Input: part model. Units: mm. Frame: model coordinates. Face numbers are marked on the shaded views. A direction names the side the tool comes from. Coordinates: 2 decimals unless noted, no trailing zeros. Order: outer loops, then holes, each group sorted by start corner. A loop starts at its lowest first (then second) coordinate and runs counter-clockwise, first axis right, second up.
Autodesk Inventor part; units mm, degrees
ref_plane "YZ Plane" through (0, 0, 0) normal (1, 0, 0) x (0, 1, 0)
ref_plane "XZ Plane" through (0, 0, 0) normal (0, 1, 0) x (-1, 0, 0)
ref_plane "XY Plane" through (0, 0, 0) normal (0, 0, 1) x (1, 0, 0)
sketch "Sketch1" plane through (0, 0, 0) normal (0, 1, 0) x (-1, 0, 0)
  line L0 (14.4237, 0) -> (-15, 0)
  line L1 (0, 25) -> (0, -25.6825)
  line L2 (6.5, 6.5) -> (-6.5, 6.5)
  line L3 (-6.5, 6.5) -> (-6.5, -6.5)
  line L4 (-6.5, -6.5) -> (6.5, -6.5)
  line L5 (6.5, -6.5) -> (6.5, 6.5)
  point P0 (0, 0)
  dimension "d0" = 13
  dimension "d1" = 0
  dimension "d10" = 0
extrude "Body" add sketch "Sketch1" along normal blind 20
sketch "Sketch2" plane through (0, 0, 0) normal (0, -1, 0) x (1, 0, 0)
  circle A0 centre (0, 0) radius 2.6
  dimension "d4" = 5.2
extrude "Screw Thread Hole" cut sketch "Sketch2" against normal through all
sketch "Sketch3" plane through (0, 20, 0) normal (0, 1, 0) x (1, 0, 0)
  line L0 (4.25, -4.25) -> (-4.25, -4.25)
  line L1 (-4.25, -4.25) -> (-4.25, 4.25)
  line L2 (-4.25, 4.25) -> (4.25, 4.25)
  line L3 (4.25, 4.25) -> (4.25, -4.25)
  line L4 (4.25, -4.25) -> (-4.25, 4.25) construction
  line L5 (-4.25, -4.25) -> (4.25, 4.25) construction
  point P0 (0, 0)
  dimension "d11" = 8.5
extrude "Connector" cut sketch "Sketch3" against normal blind 6
properties part number "Screw Port 6_8"
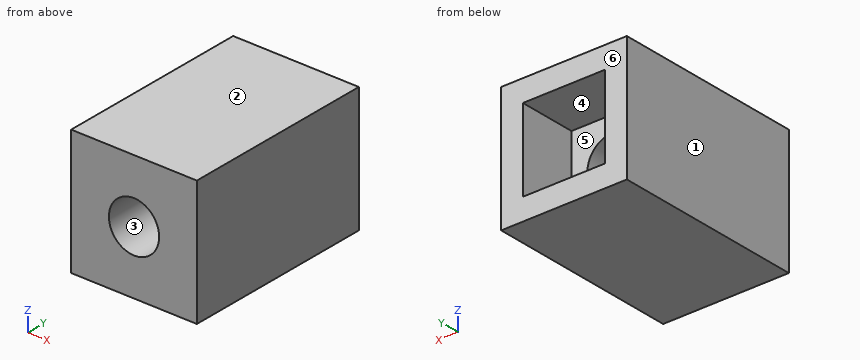
Item 1: Pin query (flat end, axial travel): pin 1 Ø4 at (x, z) = (-1.5, 0) entering from +Y. Return the tip coordinate at first contact, or that it passes through.
Response values:
pin 1: stops at y = 14
Item 2: Cut plane C-C on x = 0. Return loops of the section in (y, z), then the cut area to 3 significant figures.
Response values:
outline: (0, -6.5) - (20, -6.5) - (20, -4.25) - (14, -4.25) - (14, -2.6) - (0, -2.6) - close; (0, 2.6) - (14, 2.6) - (14, 4.25) - (20, 4.25) - (20, 6.5) - (0, 6.5) - close
area: 136 mm2
Item 3: Ray query, probe 1 along Z at (x, y) = (-1.75, 18); probe 2 along Z at (x, y) = (0, 6.25). Return the intervals inside material, ascending.
Response values:
probe 1: z = -6.5 to -4.25, 4.25 to 6.5
probe 2: z = -6.5 to -2.6, 2.6 to 6.5
Item 4: Cut plane D-D on x = 3.5. Return loops of the section in (y, z), then the cut area to 3 significant figures.
Response values:
outline: (0, -6.5) - (20, -6.5) - (20, -4.25) - (14, -4.25) - (14, 4.25) - (20, 4.25) - (20, 6.5) - (0, 6.5) - close
area: 209 mm2
Item 5: Cut plane B-B on z = 0. Return loops of the section in (x, y).
Response values:
outline: (-6.5, 0) - (-2.6, 0) - (-2.6, 14) - (-4.25, 14) - (-4.25, 20) - (-6.5, 20) - close; (2.6, 0) - (6.5, 0) - (6.5, 20) - (4.25, 20) - (4.25, 14) - (2.6, 14) - close
Item 6: Cut plane A-A on y = 14.75. Return loops of the section in (x, z).
Response values:
outline: (-6.5, -6.5) - (6.5, -6.5) - (6.5, 6.5) - (-6.5, 6.5) - close; hole (-4.25, -4.25) - (4.25, -4.25) - (4.25, 4.25) - (-4.25, 4.25) - close
Item 7: Draft query along Z for the marked faces 1, 2, 3 and 4. Return one class per face: pulls with the +Z half, pulls with the -Z half, needs draft (parallel to the pull), parting line crosses it, or undercut.
Response values:
face 1: needs draft
face 2: pulls with the +Z half
face 3: undercut
face 4: undercut
Item 8: Access query for the marked faces 5 and 6. Directions: +Z, -Z, +X, -X, +Y, -Y. A direction counts if a zero-diameter tool reaches every point of the face in a straight line with its end or side. Return the directions, or none.
Response values:
face 5: +Y
face 6: +Z, -Z, +X, -X, +Y
